Autodesk Inventor part; units mm, degrees
ref_plane "ip_cst_1_or_1_XY" through (0, 0, 0) normal (1, 0, 0) x (0, 0, -1)
ref_plane "ip_cst_1_or_1_YZ" through (0, 0, 0) normal (0, 0, -1) x (0, 1, 0)
ref_plane "ip_cst_1_or_1_ZX" through (0, 0, 0) normal (0, 1, 0) x (1, 0, 0)
sketch "Sketch_1" plane through (0, 0, 0) normal (0, 0, 1) x (1, 0, 0)
  line L0 (8, 0) -> (0, 0)
  line L1 (0, 11.5) -> (0.368, 11.5)
  line L2 (0.368, 11.5) -> (0.368, 10.75)
  line L3 (0.368, 10.75) -> (3.0318, 10.75)
  arc A0 (4.9682, 10.75) -> (3.0318, 10.75) centre (4, 9) ccw
  line L4 (4.9682, 10.75) -> (7.632, 10.75)
  line L5 (7.632, 10.75) -> (7.632, 11.5)
  line L6 (7.632, 11.5) -> (8, 11.5)
  line L7 (8, 11.5) -> (8, 12.7)
  arc A1 (8, 12.7) -> (7.7, 13) centre (7.7, 12.7) ccw
  line L8 (7.7, 13) -> (0.3, 13)
  arc A2 (0.3, 13) -> (0, 12.7) centre (0.3, 12.7) ccw
  line L9 (0, 12.7) -> (0, 11.5)
revolve "Revolution1" add sketch "Sketch_1" angle 360 about axis through (8, 0, 0) along (1, 0, 0)
ref_plane "ip_cst_1_or_1_XY" through (0, 0, 0) normal (1, 0, 0) x (0, 0, -1)
ref_plane "ip_cst_1_or_1_YZ" through (0, 0, 0) normal (0, 0, -1) x (0, 1, 0)
ref_plane "ip_cst_1_or_1_ZX" through (0, 0, 0) normal (0, 1, 0) x (1, 0, 0)
ref_plane "ip_cst_1_or_2_XY" through (0, 0, 0) normal (-1, 0, 0) x (0, 0, -1)
ref_plane "ip_cst_1_or_2_YZ" through (0, 0, 0) normal (0, 0, -1) x (0, -1, 0)
ref_plane "ip_cst_1_or_2_ZX" through (0, 0, 0) normal (0, -1, 0) x (-1, 0, 0)
ref_plane "ip_cst_1_or_3_XY" through (0.368, 0, 0) normal (1, 0, 0) x (0, 0, -1)
ref_plane "ip_cst_1_or_3_YZ" through (0.368, 0, 0) normal (0, 0, -1) x (0, 1, 0)
ref_plane "ip_cst_1_or_3_ZX" through (0.368, 0, 0) normal (0, 1, 0) x (1, 0, 0)
ref_plane "ip_cst_1_or_4_XY" through (7.632, 0, 0) normal (-1, 0, 0) x (0, 0, -1)
ref_plane "ip_cst_1_or_4_YZ" through (7.632, 0, 0) normal (0, 0, -1) x (0, -1, 0)
ref_plane "ip_cst_1_or_4_ZX" through (7.632, 0, 0) normal (0, -1, 0) x (-1, 0, 0)
properties part number "6000DDU Outer ring"
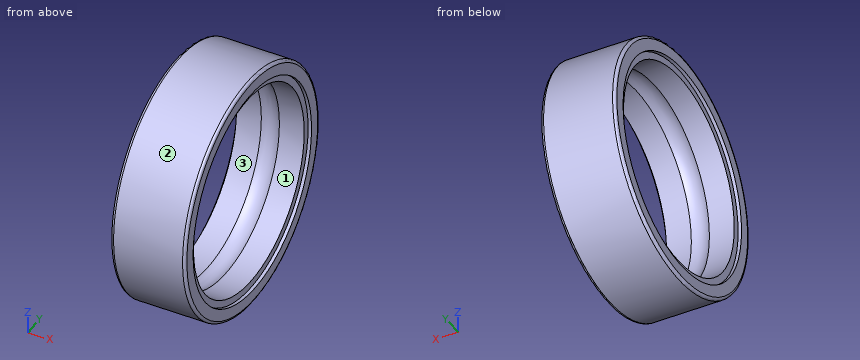
CAD build for the part. Positions are in the model's coordinates, mm. Face numbers are marked on the shaded views. Give positions to 0.01 mm unless a question says otherwise; leave off trailing zeros. Loops run counter-clockwise (first coordinate to the right, second up) from the corner with the lowest first, then second, coordinate; pieces in that order, holes last. Notation, with made-up numbers: (61, 16) -> (68, 16) arc R34 cw to (68, 49) -> close; hole circle Ø3 at (51.5, 77). An arc over 180 degrees is marked (long way). Use a Markdown table: item, result.
1. Slice it at C-C (x = 5.5). List the corners of the cut face in (y, z), plus the area to 3 significant figures.
Check result:
| item | result |
|---|---|
| outline | circle Ø26 at (0, 0); hole circle Ø21.5 at (0, 0) |
| area | 168 mm^2 |
2. Flat gauge pin, fed straight in: pin 1 (7 mm diameter, centred on y = -3, z = 4, fed in from +X). Where does the tip first touch, or does it go through?
Check result:
| item | result |
|---|---|
| pin 1 | passes through |
3. Mould opens along Y. For the marked faces 1, 2 and 3 say: pulls with the +Y half, pulls with the -Y half, needs draft (parallel to the pull), parting line crosses it, or undercut.
Check result:
| item | result |
|---|---|
| face 1 | undercut |
| face 2 | parting line crosses it |
| face 3 | undercut |
4. Slice it at A-A (z = 0). List the corners of the cut face in (x, y).
Check result:
| item | result |
|---|---|
| outline | (0, -12.7) arc R0.3 ccw to (0.3, -13) -> (7.7, -13) arc R0.3 ccw to (8, -12.7) -> (8, -11.5) -> (7.63, -11.5) -> (7.63, -10.75) -> (4.97, -10.75) arc R2 cw to (3.03, -10.75) -> (0.37, -10.75) -> (0.37, -11.5) -> (0, -11.5) -> close; (0, 11.5) -> (0.37, 11.5) -> (0.37, 10.75) -> (3.03, 10.75) arc R2 cw to (4.97, 10.75) -> (7.63, 10.75) -> (7.63, 11.5) -> (8, 11.5) -> (8, 12.7) arc R0.3 ccw to (7.7, 13) -> (0.3, 13) arc R0.3 ccw to (0, 12.7) -> close |
5. Wall check: L1, parallel to Z at x = 7.25, y = 0; L2, parallel to Z at x = 0.3, y = 0; L3, parallel to Y at x = 7, z = -8.25. Give the ranges that are in metal, low to high. Write a range as [from, to].
Check result:
| item | result |
|---|---|
| L1 | z = [-13, -10.75], [10.75, 13] |
| L2 | z = [-13, -11.5], [11.5, 13] |
| L3 | y = [-10.05, -6.89], [6.89, 10.05] |
